Read the model definition and answer for the solid it produces. Units are mm, in the model's axes. A direction names the side the tool comes from. Coordinates: 2 decimals unless noted, no trailing zeros. Loops run counter-clockwise (first coordinate to the right, second up) from the corner with the lowest first, then second, coordinate; pieces in that order, holes last.
from build123d import *

# Parameters (mm, degrees)
F0_R     = 2.5
F1_DEPTH = 8
F2_R     = 0.5
F3_R     = 1
F4_DEPTH = 12.5


with BuildPart() as f1:
    # F0 (on Top) → F1 (new body)
    with BuildSketch(Plane.XY):
        with BuildLine():
            ThreePointArc((-3.9878581514, -8.6885720566), (-2.7160898573, -6.0635300296), (0, -5))
            Line((0, -5), (2.8, -5))
            ThreePointArc((2.8, -5), (5.6284271247, -3.8284271247), (6.8, -1))
            Line((6.8, -1), (6.8, 4.1070405464))
            ThreePointArc((6.8, 4.1070405464), (7.6768943744, 6.9354676711), (10, 8.7718020623))
            Line((10, 8.7718020623), (10, 12.5))
            Line((10, 12.5), (3.1224989992, 12.5))
            ThreePointArc((3.1224989992, 12.5), (0.4005785985, 11.0201084454), (-2.5616621646, 11.9278855889))
            add(Edge.make_bspline(
                [(-6.9689841618, -1.5710293014), (-8.0102303747, 0.7595881395), (-5.9806638587, 8.3334675363), (-4.0694582276, 9.7266677767), (-2.5616621646, 11.9278855889)],
                knots=[0, 0, 0, 0, 0.5567053674, 1, 1, 1, 1], degree=3))
            ThreePointArc((-6.9689841618, -1.5710293014), (-5.7970541621, -4.324632576), (-6.8636587821, -7.1207201108))
            ThreePointArc((-6.8636587821, -7.1207201108), (-5.5019929053, -8.0444775564), (-3.9878581514, -8.6885720566))
        make_face()
        Circle(F0_R, mode=Mode.SUBTRACT)
    extrude(amount=F1_DEPTH)

    # F2
    f2_edges = [f1.edges().sort_by_distance(p)[0] for p in [
        (10, 12.5, 4),
        (3.122499, 12.5, 4),
        (-2.561662, 11.927886, 4),
        (10, 8.771802, 4),
        (-3.987858, -8.688572, 4),
        (-6.863659, -7.12072, 4),
    ]]
    fillet(f2_edges, radius=F2_R)

    # F3 (on Right) → F4 (cut, symmetric)
    with BuildSketch(Plane.YZ):
        with Locations((0, 4)):
            Circle(F3_R)
    extrude(amount=F4_DEPTH, both=True, mode=Mode.SUBTRACT)


solid = f1.part
Item 1: Find the intervals of material crossed by line 1 along Y through (x, z) = (5.55, 4); line 2 along Z through (x, y) = (-6.05, 0); line 3 along Y through (x, z) = (-2.25, 6.75), in increasing order.
Numbers:
line 1: y = -3.9 to -1, 1 to 12.5
line 2: z = 0 to 3, 5 to 8
line 3: y = -5.69 to -1.09, 1.09 to 11.68
Item 2: Which of the six approach directions +Z, -Z, +X, -X, +Y, -Y give full straight-line access (tool end or side, diameter ignored) to faces 4 (the face through (6.8, 2, 4)), 5 (the face through (5, 0, 5))?
Numbers:
face 4: +Z, -Z, +X, -Y
face 5: +X, -X
Item 3: A cutting plane is placed at A-A on x = -1.5. Determine the outline of the cut face in (y, z).
Numbers:
outline: (-5.29, 0) - (-2, 0) - (-2, 8) - (-5.29, 8) - close; (2, 0) - (11.29, 0) - (11.29, 8) - (2, 8) - close
Item 4: Determine the mould class of faces 1 (the face through (0.57, 11.04, 3.94)), 2 (the face through (1.15, -2.22, 3.94)), 3 (the face through (1, 4, 0)) for opening direction Y: released by +Y, released by -Y, zero draft, split by the parting line, or undercut.
Numbers:
face 1: released by +Y
face 2: undercut
face 3: zero draft
Item 5: Given pin 1 (2.5 mm diameter, centred on y = 0, z = 4, fed in from +X); pin 2 (2 mm diameter, centred on y = 5.5, z = 6.5, fed in from +X); pin 3 (1.6 mm diameter, centred on y = 0, z = 4, fed in from +X); pin 4 (2 mm diameter, centred on x = 1, z = 4.5, fed in from -Y), each flat-ended and moving along its own axis, determine where each tip first touches the part or whether it passes through.
Numbers:
pin 1: stops at x = 6.8
pin 2: stops at x = 7.41
pin 3: passes through
pin 4: stops at y = -5
Item 6: A cutting plane is placed at D-D on y = -3.25. Determine the outline of the cut face in (x, z).
Numbers:
outline: (-5.97, 0) - (6.11, 0) - (6.11, 8) - (-5.97, 8) - close
Item 7: A cutting plane is placed at C-C on x = 8.25. Determine the outline of the cut face in (y, z).
Numbers:
outline: (7.63, 0) - (12.5, 0) - (12.5, 8) - (7.63, 8) - close
Item 8: A cutting plane is placed at B-B on y = -0.5. Give the number of separate pieces and of enclosed holes in the cut face, then the cut area to 3 significant figures.
Numbers:
separate pieces: 4
enclosed holes: 0
area: 57.6 mm2
